Geometry: see drawing. Coordinates: mm, zero at the bounding-box minimum. Coordinates: 2 decimals unless noted, no trailing zeros. Loops run counter-clockwise (first coordinate to the right, second up) from the corner with the lowest first, then second, coordinate; pieces in that order, holes last. Notation, with made-up numbers: (-37.5, -10) - (-25.5, -10) arc R10 ccw to (-25.5, 9) - close; hole circle Ø8 at (4.25, -36). An arc over 180 degrees is marked (long way). Use one line per item in the form item = value.
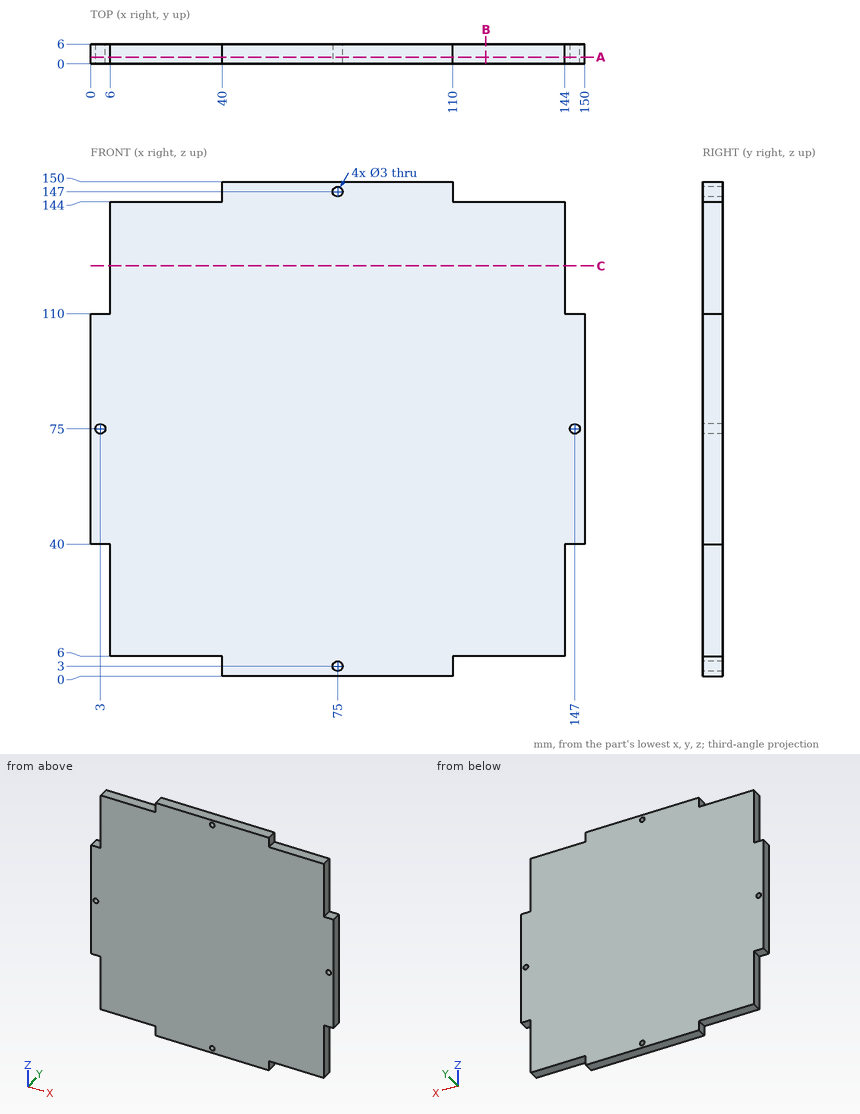
Q1. First-contact query: P1, Ø1.8, axis at x = 135.5, y = 3, coming from the +Z side; P2, Ø1.8, axis at y = 4.5, z = 146, coming from the -X side; P3, Ø1.8, axis at x = 132.5, y = 4, coming from the -Z side. Flat tips, straight axial feed; report the tip coordinate or a pass-through.
Check values:
P1 = 144
P2 = 40
P3 = 6
Q2. Cut plane C-C, the plane z = 124.5. Return loops of the section in (x, y).
Check values:
outline = (6, 0) - (144, 0) - (144, 6) - (6, 6) - close
Q3. Cut plane A-A, the plane y = 2. Return loops of the section in (x, z).
Check values:
outline = (0, 40) - (6, 40) - (6, 6) - (40, 6) - (40, 0) - (110, 0) - (110, 6) - (144, 6) - (144, 40) - (150, 40) - (150, 110) - (144, 110) - (144, 144) - (110, 144) - (110, 150) - (40, 150) - (40, 144) - (6, 144) - (6, 110) - (0, 110) - close; hole circle Ø3 at (3, 75); hole circle Ø3 at (75, 3); hole circle Ø3 at (75, 147); hole circle Ø3 at (147, 75)
Q4. Ray query, line 1 along Z through (x, y) = (75, 1.8); line 2 along X through (y, z) = (2.85, 147). Return the intervals inside material, ascending. Write a range as [from, to].
Check values:
line_1 = [0, 1.5], [4.5, 145.5], [148.5, 150]
line_2 = [40, 73.5], [76.5, 110]
Q5. Cut plane B-B, the plane x = 120. Return loops of the section in (y, z).
Check values:
outline = (0, 6) - (6, 6) - (6, 144) - (0, 144) - close
